Read the model definition and answer for the solid it produces. Units are mm, in the model's axes. Coordinates: 2 decimals unless noted, no trailing zeros. Order: outer loops, then holes, each group sorted by start corner. A loop starts at its lowest first (then second) coordinate and runs counter-clockwise, first axis right, second up.
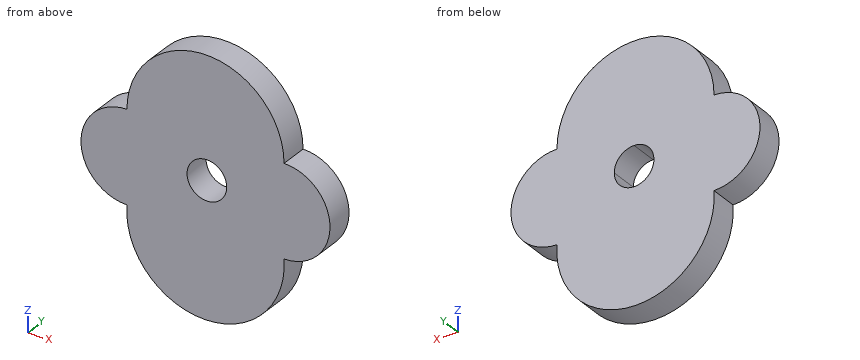
from build123d import *

# Parameters (mm, degrees)
F1_DEPTH = 25.4


with BuildPart() as f1:
    # F0 (on Front) → F1 (new body)
    with BuildSketch(Plane.XZ):
        with BuildLine():
            ThreePointArc((69.7280094028, 37.8677658737), (-1.2611225247, 108.8568978012), (-72.2502544522, 37.8677658737))
            Line((-72.2502544522, 37.8677658737), (-51.3892844319, 37.8677658737))
            Line((-51.3892844319, 37.8677658737), (0, 37.8677658737))
            Line((0, 37.8677658737), (69.7280094028, 37.8677658737))
        make_face()
        Polygon((-51.3892844319, 37.8677658737), (-72.2502544522, 37.8677658737), (-72.2502544522, -45.2175028622), (69.7280094028, -45.2175028622), (69.7280094028, -29.6100229025), (-51.3892844319, -29.6100229025), align=None)
        with BuildLine():
            Line((-72.2502544522, -45.2175028622), (-72.2502544522, 37.8677658737))
            ThreePointArc((-72.2502544522, 37.8677658737), (-113.7928888202, -3.6748684943), (-72.2502544522, -45.2175028622))
        make_face()
        with BuildLine():
            Line((0, 37.8677658737), (-51.3892844319, 37.8677658737))
            Line((-51.3892844319, 37.8677658737), (-51.3892844319, -29.6100229025))
            Line((-51.3892844319, -29.6100229025), (69.7280094028, -29.6100229025))
            Line((69.7280094028, -29.6100229025), (69.7280094028, 0))
            Line((69.7280094028, 0), (17.9303269799, 0))
            ThreePointArc((17.9303269799, 0), (-12.6786557964, -12.6786557964), (0, 17.9303269799))
            Line((0, 17.9303269799), (0, 37.8677658737))
        make_face()
        with BuildLine():
            Line((69.7280094028, -45.2175028622), (-72.2502544522, -45.2175028622))
            ThreePointArc((-72.2502544522, -45.2175028622), (-1.2611225247, -121.5592398304), (69.7280094028, -45.2175028622))
        make_face()
        with BuildLine():
            Line((69.7280094028, 0), (69.7280094028, 37.8677658737))
            Line((69.7280094028, 37.8677658737), (0, 37.8677658737))
            Line((0, 37.8677658737), (0, 17.9303269799))
            ThreePointArc((0, 17.9303269799), (12.6786557964, 12.6786557964), (17.9303269799, 0))
            Line((17.9303269799, 0), (69.7280094028, 0))
        make_face()
        with BuildLine():
            ThreePointArc((69.7280094028, -45.2175028622), (111.2706437707, -3.6748684943), (69.7280094028, 37.8677658737))
            Line((69.7280094028, 37.8677658737), (69.7280094028, 0))
            Line((69.7280094028, 0), (69.7280094028, -29.6100229025))
            Line((69.7280094028, -29.6100229025), (69.7280094028, -45.2175028622))
        make_face()
    extrude(amount=F1_DEPTH)


solid = f1.part
Q1. The part is cut by section C-C, the plane z = -26.5. Determine the outline of the cut face in (x, y), then the cut area to 3 significant figures.
Q2. The part is cut by section D-D, the plane z = 72.5. Determine the outline of the cut face in (x, y), then the cut area to 3 significant figures.
Q3. The part is cut by section B-B, the plane y = -4.5. Determine the outline of the cut face in (x, z).
Q4. The part is cut by section A-A, the plane x = 9.5. Determine the outline of the cut face in (y, z), then the cut area to 3 significant figures.
Q5. Straight lines are drawn through the part: L1, parallel to Z at x = -15.5, y = -6.5; L2, parallel to X at y = -10.75, z = 0; L3, parallel to X at y = -10.5, z = 4. For each, find the intervals that lie inside material, in ascending order.
Q6. Each of these flat-tipped pins is pushed along its axis until it touches: P1, Ø6, axis at y = -3.5, z = 69, coming from the +X side; P2, Ø12, axis at y = -21.5, z = 35.5, coming from the -X side; P3, Ø8, axis at y = -6, z = 28, coming from the -X side. Where does it stop, or does it pass through?
Computed values:
1. outline: (-106.96, -25.4) - (104.44, -25.4) - (104.44, 0) - (-106.96, 0) - close
1. area: 5,370 mm2
2. outline: (-63.23, -25.4) - (60.71, -25.4) - (60.71, 0) - (-63.23, 0) - close
2. area: 3,150 mm2
3. outline: (-72.25, -45.22) arc R71.18 ccw (long way) to (69.73, -45.22) arc R41.54 ccw to (69.73, 37.87) arc R70.99 ccw to (-72.25, 37.87) arc R41.54 ccw to start; hole circle Ø35.86 at (0, 0)
4. outline: (-25.4, -120.74) - (0, -120.74) - (0, -15.21) - (-25.4, -15.21) - close; (-25.4, 15.21) - (0, 15.21) - (0, 108.04) - (-25.4, 108.04) - close
4. area: 5,040 mm2
5. L1: z = -120.12 to -9.01, 9.01 to 107.41
5. L2: x = -113.63 to -17.93, 17.93 to 111.11
5. L3: x = -113.08 to -17.48, 17.48 to 110.56
6. P1: stops at x = 63.92
6. P2: stops at x = -97.25
6. P3: stops at x = -103.23
